Answer from the drawing. Dimensions are ordinates in mm from the lowest x, y and z of the part. Give positions to 0.01 mm unless a question says otherwise; leave off trailing zeros. Order: outer loops, then holes, each group sorted by start corner. A loop starts at its lowest first (then second) coordinate and runs counter-clockwise, first axis right, second up.
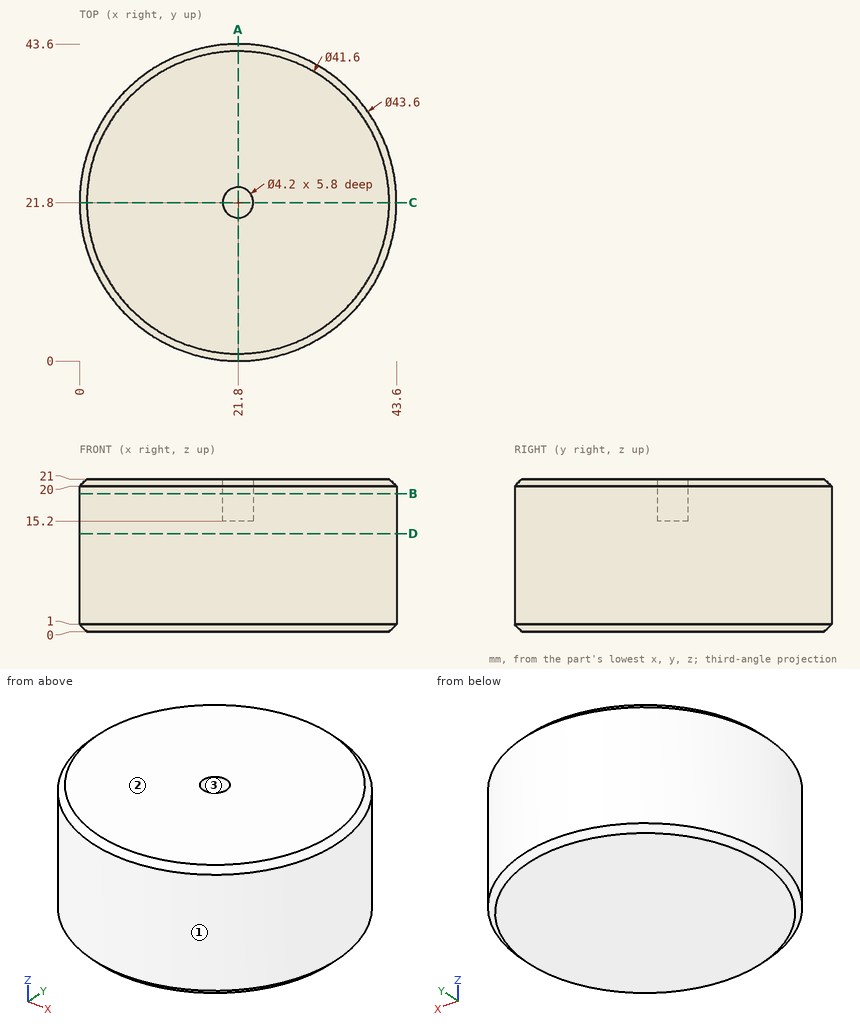
1. The part is cut by section A-A (x = 21.8). Write down the section's boundary in (y, z).
Findings below:
outline: (0, 1) - (1, 0) - (42.6, 0) - (43.6, 1) - (43.6, 20) - (42.6, 21) - (23.9, 21) - (23.9, 15.2) - (19.7, 15.2) - (19.7, 21) - (1, 21) - (0, 20) - close
2. The mould has two halves that part along X. Classify the marked faces 1, 2 and 3: pulls with the +X half, pulls with the -X half, needs draft (parallel to the pull), parting line crosses it, or undercut.
Findings below:
face 1: parting line crosses it
face 2: needs draft
face 3: undercut
3. Given P1, Ø3, axis at x = 26.5, z = 11, coming from the -Y side; P2, Ø12, axis at y = 15.5, z = 14.5, coming from the -X side; P3, Ø2, axis at x = 22.5, y = 22, coming from the +Z side, each flat-ended and moving along its own axis, determine where each tip first touches the part or whether it passes through.
Findings below:
P1: stops at y = 0.24
P2: stops at x = 0
P3: stops at z = 15.2
4. The part is cut by section D-D (z = 13.5). Write down the section's boundary in (x, y), then the cut area to 3 significant figures.
Findings below:
outline: circle Ø43.6 at (21.8, 21.8)
area: 1,490 mm2
5. The part is cut by section B-B (z = 19). Write down the section's boundary in (x, y), then the cut area to 3 significant figures.
Findings below:
outline: circle Ø43.6 at (21.8, 21.8); hole circle Ø4.2 at (21.8, 21.8)
area: 1,480 mm2
6. Straight lines are drawn through the part: probe 1 along Y at (x, z) = (21.8, 16.45); probe 2 along Y at (x, z) = (21.5, 9); probe 3 along Y at (x, z) = (26.5, 8.5). For each, find the intervals that lie inside material, in ascending order.
Findings below:
probe 1: y = 0 to 19.7, 23.9 to 43.6
probe 2: y = 0 to 43.6
probe 3: y = 0.51 to 43.09
